Can you work these out from the model? Positions are in its coordinate system, mm. Give positions to 0.01 mm unless a question says otherwise; leave off trailing zeros.
Item 1: I want a section at A-A, the plane y = 157.5. Count the separate pieces of the cut face and the enclosed holes in it, then the cut area to 3 significant figures.
Item 2: I'm going to push a flat-ended pin straight in: pin 1 Ø1 at (x, z) = (86.5, 1.5) entering from -Y. Where does the tip first touch, or does it pass through?
Item 3: If I drill on line 1 along Y through (x, z) = (78.5, 2.45), over which ranges is the centre line in solid material (lowest first)?
```python
from build123d import *

# Parameters (mm, degrees)
SKETCH1_W           = 133.35
SKETCH1_H           = 254
BOSS_EXTRUDE1_DEPTH = 3.175
SKETCH2_W           = 6.35
SKETCH2_H           = 150
CUT_EXTRUDE1_DEPTH  = 3.175


with BuildPart() as part:
    # Sketch1 → Boss-Extrude1 (new body)
    with BuildSketch(Plane.XY):
        with Locations((66.675, 127)):
            Rectangle(SKETCH1_W, SKETCH1_H)
    extrude(amount=BOSS_EXTRUDE1_DEPTH)

    # Sketch2 → Cut-Extrude1 (cut)
    with BuildSketch(Plane.XY.offset(3.175)):
        with Locations((19.05, 85)):
            Rectangle(SKETCH2_W, SKETCH2_H)
        with Locations((28.58, 85)):
            Rectangle(SKETCH2_W, SKETCH2_H)
        with Locations((38.11, 85)):
            Rectangle(SKETCH2_W, SKETCH2_H)
        with Locations((47.64, 85)):
            Rectangle(SKETCH2_W, SKETCH2_H)
        with Locations((57.17, 85)):
            Rectangle(SKETCH2_W, SKETCH2_H)
        with Locations((66.7, 85)):
            Rectangle(SKETCH2_W, SKETCH2_H)
        with Locations((76.23, 85)):
            Rectangle(SKETCH2_W, SKETCH2_H)
        with Locations((85.76, 85)):
            Rectangle(SKETCH2_W, SKETCH2_H)
        with Locations((95.29, 85)):
            Rectangle(SKETCH2_W, SKETCH2_H)
        with Locations((104.82, 85)):
            Rectangle(SKETCH2_W, SKETCH2_H)
        with Locations((114.35, 85)):
            Rectangle(SKETCH2_W, SKETCH2_H)
    extrude(amount=-CUT_EXTRUDE1_DEPTH, mode=Mode.SUBTRACT)


solid = part.part
```
Results list:
1. separate pieces: 12
1. enclosed holes: 0
1. area: 202 mm2
2. pin 1: stops at y = 0
3. line 1: y = 0 to 10, 160 to 254
